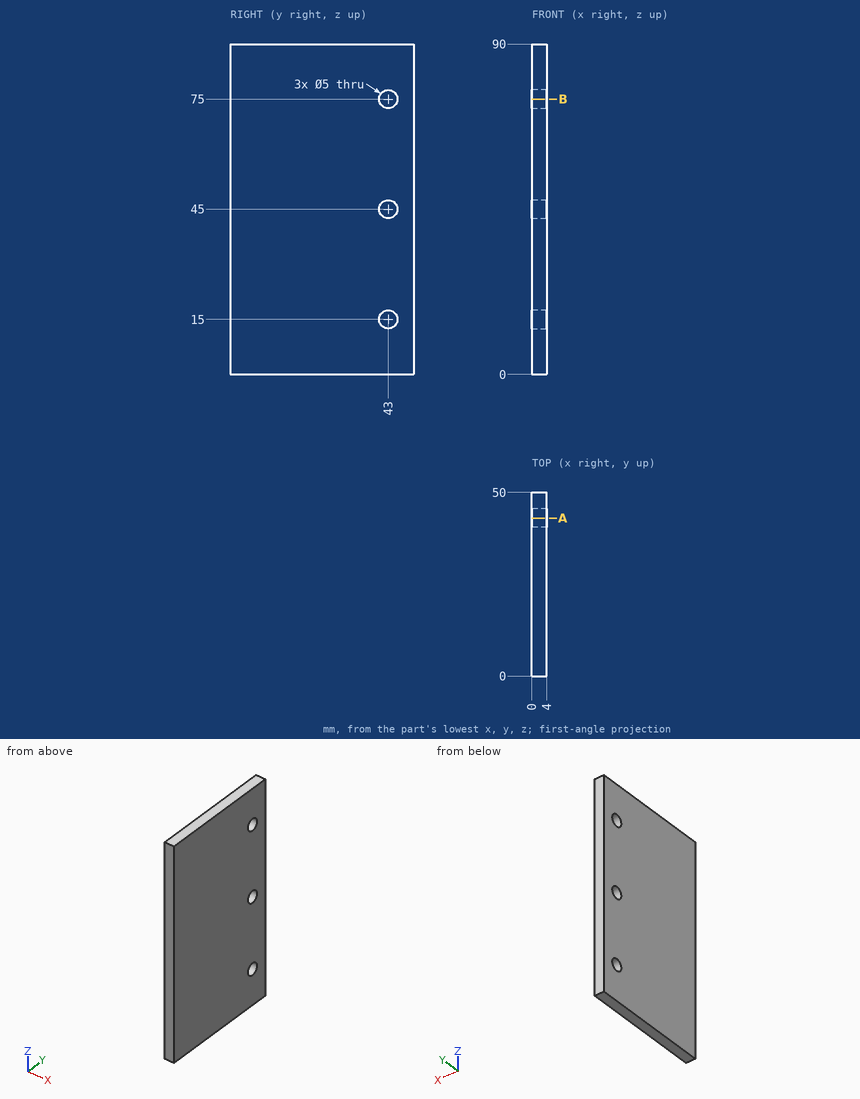
Drawing for the job (mm, zero at the part's lowest x, y, z). Coordinates: 2 decimals unless noted, no trailing zeros. Order: outer loops, then holes, each group sorted by start corner. A loop starts at its lowest first (then second) coordinate and runs counter-clockwise, first axis right, second up. Notation, with made-up numbers: (-4, 32) - (19, 32) arc R18 ccw to (19, 59) - close; hole circle Ø11 at (87, 45.5). An arc over 180 degrees is marked (long way). Use a Markdown table: item, result. Add a question column.
(1) Drill centre lines: line 1 along Z through (x, y) = (1.85, 43); line 2 along Y through (x, z) = (3.15, 75); line 3 along Z through (x, y) = (2.1, 45). Where is each one in solid material? Low to high. Write a range as [from, to].
(2) Saw through at B-B (z = 75). Give the cut face in (x, y).
(3) Flat gauge pin, fed straight in: pin 1 (4 mm diameter, centred on y = 43, z = 75, fed in from -X). Where does the tip first touch, or does it go through?
(4) Saw through at A-A (y = 43). Give the cut face in (x, z).
Solved:
| question | item | result |
|---|---|---|
| 1 | line 1 | z = [0, 12.5], [17.5, 42.5], [47.5, 72.5], [77.5, 90] |
| 1 | line 2 | y = [0, 40.5], [45.5, 50] |
| 1 | line 3 | z = [0, 13.5], [16.5, 43.5], [46.5, 73.5], [76.5, 90] |
| 2 | outline | (0, 0) - (4, 0) - (4, 40.5) - (0, 40.5) - close; (0, 45.5) - (4, 45.5) - (4, 50) - (0, 50) - close |
| 3 | pin 1 | passes through |
| 4 | outline | (0, 0) - (4, 0) - (4, 12.5) - (0, 12.5) - close; (0, 17.5) - (4, 17.5) - (4, 42.5) - (0, 42.5) - close; (0, 47.5) - (4, 47.5) - (4, 72.5) - (0, 72.5) - close; (0, 77.5) - (4, 77.5) - (4, 90) - (0, 90) - close |
